Autodesk Fusion 360 part; units mm, degrees
sketch "Sketch1" plane through (0, 0, 0) normal (0, 0, 1) x (1, 0, 0)
  line L0 (390.525, -352) -> (-390.525, -352)
  line L1 (-390.525, -352) -> (-390.525, 352)
  line L2 (-390.525, 352) -> (390.525, 352)
  line L3 (390.525, 352) -> (390.525, -352)
  line L4 (390.525, -352) -> (-390.525, 352) construction
  line L5 (-390.525, -352) -> (390.525, 352) construction
  circle A0 centre (0, 0) radius 10
  circle A1 centre (-288, -288) radius 10
  circle A2 centre (-192, -288) radius 10
  circle A3 centre (-96, -288) radius 10
  circle A4 centre (0, -288) radius 10
  circle A5 centre (96, -288) radius 10
  circle A6 centre (192, -288) radius 10
  circle A7 centre (288, -288) radius 10
  circle A8 centre (-288, -192) radius 10
  circle A9 centre (-192, -192) radius 10
  circle A10 centre (-96, -192) radius 10
  circle A11 centre (0, -192) radius 10
  circle A12 centre (96, -192) radius 10
  circle A13 centre (192, -192) radius 10
  circle A14 centre (288, -192) radius 10
  circle A15 centre (-288, -96) radius 10
  circle A16 centre (-192, -96) radius 10
  circle A17 centre (-96, -96) radius 10
  circle A18 centre (0, -96) radius 10
  circle A19 centre (96, -96) radius 10
  circle A20 centre (192, -96) radius 10
  circle A21 centre (288, -96) radius 10
  circle A22 centre (-288, 0) radius 10
  circle A23 centre (-192, 0) radius 10
  circle A24 centre (-96, 0) radius 10
  circle A25 centre (96, 0) radius 10
  circle A26 centre (192, 0) radius 10
  circle A27 centre (288, 0) radius 10
  circle A28 centre (-288, 96) radius 10
  circle A29 centre (-192, 96) radius 10
  circle A30 centre (-96, 96) radius 10
  circle A31 centre (0, 96) radius 10
  circle A32 centre (96, 96) radius 10
  circle A33 centre (192, 96) radius 10
  circle A34 centre (288, 96) radius 10
  circle A35 centre (-288, 192) radius 10
  circle A36 centre (-192, 192) radius 10
  circle A37 centre (-96, 192) radius 10
  circle A38 centre (0, 192) radius 10
  circle A39 centre (96, 192) radius 10
  circle A40 centre (192, 192) radius 10
  circle A41 centre (288, 192) radius 10
  circle A42 centre (-288, 288) radius 10
  circle A43 centre (-192, 288) radius 10
  circle A44 centre (-96, 288) radius 10
  circle A45 centre (0, 288) radius 10
  circle A46 centre (96, 288) radius 10
  circle A47 centre (192, 288) radius 10
  circle A48 centre (288, 288) radius 10
  circle A49 centre (384, -288) radius 10
  circle A50 centre (384, -192) radius 10
  circle A51 centre (384, -96) radius 10
  circle A52 centre (384, 0) radius 10
  circle A53 centre (384, 96) radius 10
  circle A54 centre (384, 192) radius 10
  circle A55 centre (384, 288) radius 10
  dimension "d1" = 781.05
  dimension "d2" = 704
  dimension "d3" = 20
  dimension "d6" = 96
  dimension "d7" = 96
extrude "Extrude1" add sketch "Sketch1" along normal blind 19.05 contours L0 L1 L2 L3 A49 A50 A51 A52 A53 A54 A55 | L3 A49 | L3 A50 | L3 A55 | L3 A51 | L3 A54 | L3 A52 | L3 A53 picked at (384.7263, -291.1646) picked at (379.6291, -189.2794) picked at (384.7263, 284.8354) picked at (385.0976, -95.2699) picked at (388.2662, 188.6677) picked at (386.0356, -2.4329) picked at (385.0976, 95.2699)
sketch "Sketch2" plane through (0, 0, 19.05) normal (0, 0, 1) x (-1, 0, 0)
  circle A0 centre (192, -288) radius 10
  circle A1 centre (-192, -288) radius 10
  circle A2 centre (96, 192) radius 10
  circle A3 centre (288, 192) radius 10
  circle A4 centre (0, 192) radius 10
  circle A5 centre (288, 96) radius 10
  circle A6 centre (96, 0) radius 10
  circle A7 centre (288, 0) radius 10
  circle A8 centre (192, 0) radius 10
  circle A9 centre (-192, 0) radius 10
  circle A10 centre (-288, 0) radius 10
  circle A11 centre (288, -96) radius 10
  circle A12 centre (-96, 0) radius 10
  circle A13 centre (-96, -288) radius 10
  circle A14 centre (192, 192) radius 10
  circle A15 centre (-288, -288) radius 10
  circle A16 centre (0, -288) radius 10
  circle A17 centre (-288, -192) radius 10
  circle A18 centre (192, -192) radius 10
  circle A19 centre (96, -192) radius 10
  circle A20 centre (288, -192) radius 10
  circle A21 centre (-288, -96) radius 10
  circle A22 centre (0, -96) radius 10
  circle A23 centre (-96, -96) radius 10
  circle A24 centre (-192, -96) radius 10
  circle A25 centre (-192, -192) radius 10
  circle A26 centre (-96, 96) radius 10
  circle A27 centre (-288, 96) radius 10
  circle A28 centre (-192, 96) radius 10
  circle A29 centre (0, 96) radius 10
  circle A30 centre (96, 96) radius 10
  circle A31 centre (192, 96) radius 10
  circle A32 centre (-96, 192) radius 10
  circle A33 centre (-192, 192) radius 10
  circle A34 centre (-288, 192) radius 10
  circle A35 centre (192, -96) radius 10
  circle A36 centre (288, -288) radius 10
  circle A37 centre (96, -96) radius 10
  circle A38 centre (96, -288) radius 10
  circle A39 centre (-96, -192) radius 10
  circle A40 centre (288, 288) radius 10
  circle A41 centre (-96, 288) radius 10
  circle A42 centre (192, 288) radius 10
  circle A43 centre (-192, 288) radius 10
  circle A44 centre (0, 0) radius 10
  circle A45 centre (0, 288) radius 10
  circle A46 centre (-288, 288) radius 10
  circle A47 centre (0, -192) radius 10
  circle A48 centre (96, 288) radius 10
  line L0 (-390.525, -352) -> (390.525, -352)
  line L1 (390.525, -352) -> (390.525, 352)
  line L2 (390.525, 352) -> (-390.525, 352)
  line L3 (-390.525, 352) -> (-390.525, -352)
  point P0 (363.525, -325)
  point P1 (0.025, -325)
  point P2 (-363.475, -325)
  point P3 (363.525, 0)
  point P4 (0.025, 0)
  point P5 (-363.475, 0)
  point P6 (363.525, 325)
  point P7 (0.025, 325)
  point P8 (-363.475, 325)
  dimension "d17" = 27
  dimension "d18" = 27
  dimension "d21" = 727
  dimension "d22" = 650
hole "Hole1" at (-363.525, 325, 19.05) at (-0.025, 325, 19.05) at (-363.525, 0, 19.05) at (-363.525, -325, 19.05) at (-0.025, -325, 19.05) at (363.475, -325, 19.05) at (363.475, 0, 19.05) at (363.475, 325, 19.05) direction (0, 0, -1) diameter 6.35 end through all counterbore diameter 19.05 counterbore depth 9.8425
equation "d8 = ( 3 / 4 ) * 1 in"
Input: part model. Units: mm. Frame: model coordinates. A direction names the side the tool comes from. Give positions to 0.01 mm unless a question says otherwise; leave off trailing zeros.
Q1. Pull-direction query (X, two-part tool) for faces 3 (the face through (-5, -73, 19.05)), 4 (the face through (354.03, 326.24, 14.06)), 5 (the face through (390.525, 5, 9)); classes: pulls with the +X half, pulls with the -X half, needs draft (parallel to the pull), parting line crosses it, or undercut.
Q2. Material intervals for probe 1 along X at (y, z) = (-325, 11.5) (3 decimals), sorted ascending.
Q3. Set-up query: faces 1 (the face through (-98.17, 297.76, 9.39)), 2 (the face through (-372.97, 1.24, 14.06)). Return all of +Z, -Z, +X, -X, +Y, -Y with unobstructed straight access to the full face (end or side cutting, diameter ignored); none if empty.
Q4. Section A-A, the plane y = -96. State how many separate pieces and enclosed holes the cut face has, plus the area to 3 significant figures.
Filled in:
1. face 3: needs draft
1. face 4: undercut
1. face 5: pulls with the +X half
2. probe 1: x = -390.525 to -373.05, -354 to -9.55, 9.5 to 353.95, 373 to 390.525
3. face 1: +Z, -Z
3. face 2: +Z
4. separate pieces: 8
4. enclosed holes: 0
4. area: 12,200 mm2
